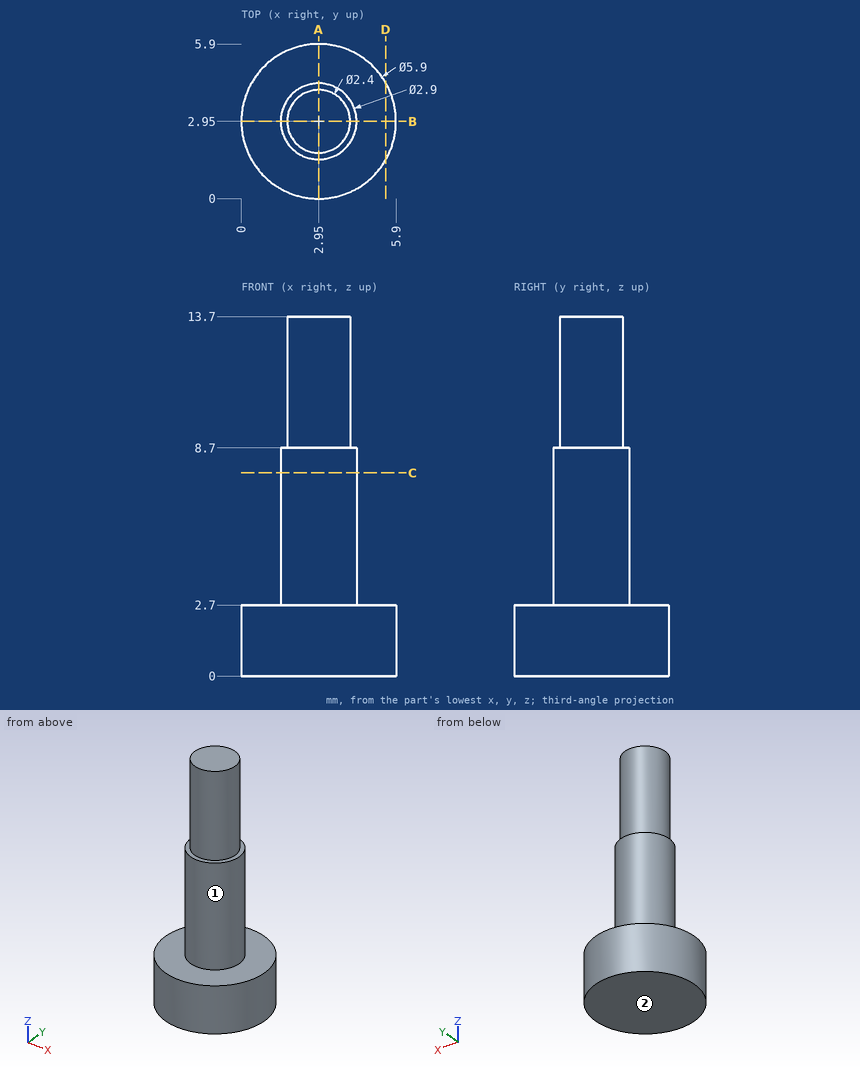
Verification items for this drawing (mm, ordinates from the low corner). A direction names the side the tool comes from. Round coordinates to 2 decimals unless told otherwise and drop trailing zeros. Loops run counter-clockwise (first coordinate to the right, second up) from the corner with the lowest first, then second, coordinate; pieces in that order, holes last. Notation, with made-up numbers: (79.5, -17.75) -> (109.5, -17.75) arc R18 ccw to (109.5, 3.25) -> close; hole circle Ø11 at (24.25, 8). An arc over 180 degrees is marked (long way). Answer in a Markdown table with one row per item.
Q1. Thickness scan on L1, parallel to Z at x = 3.05, y = 0.7; L2, parallel to X at y = 3, z = 12; L3, parallel to Z at x = 4.3, y = 2.6. Record the ranges inside material, lowest first.
Data:
| item | result |
|---|---|
| L1 | z = 0 to 2.7 |
| L2 | x = 1.75 to 4.15 |
| L3 | z = 0 to 8.7 |
Q2. Sectioned sample at C-C on z = 7.75. Enter the section's corners in (x, y), then the cut area to 3 significant figures.
Data:
| item | result |
|---|---|
| outline | circle Ø2.9 at (2.95, 2.95) |
| area | 6.61 mm^2 |
Q3. Set-up check for the marked faces 1 and 2: record each of +Z, -Z, +X, -X, +Y, -Y from which the full face is reachable in a straight line by a thin tool's end or side.
Data:
| item | result |
|---|---|
| face 1 | +Z |
| face 2 | -Z, +X, -X, +Y, -Y |
Q4. Go/stop test with flat-tipped pins: P1, Ø3, axis at x = 4, z = 5.5, coming from the +Y side; P2, Ø1, axis at y = 2, z = 10.5, coming from the +X side; P3, Ø3, axis at x = 2.5, y = 1, coming from the +Z side; P4, Ø1.5, axis at x = 2, y = 1, coming from the +Z side. Record where each tip stops, or that it passes through.
Data:
| item | result |
|---|---|
| P1 | stops at y = 4.4 |
| P2 | stops at x = 4.06 |
| P3 | stops at z = 13.7 |
| P4 | stops at z = 8.7 |
Q5. Sectioned sample at D-D on x = 5.5. Enter the section's corners in (y, z).
Data:
| item | result |
|---|---|
| outline | (1.47, 0) -> (4.43, 0) -> (4.43, 2.7) -> (1.47, 2.7) -> close |
Q6. Sectioned sample at A-A on x = 2.95. Enter the section's corners in (y, z), then the cut area to 3 significant figures.
Data:
| item | result |
|---|---|
| outline | (0, 0) -> (5.9, 0) -> (5.9, 2.7) -> (4.4, 2.7) -> (4.4, 8.7) -> (4.15, 8.7) -> (4.15, 13.7) -> (1.75, 13.7) -> (1.75, 8.7) -> (1.5, 8.7) -> (1.5, 2.7) -> (0, 2.7) -> close |
| area | 45.3 mm^2 |
